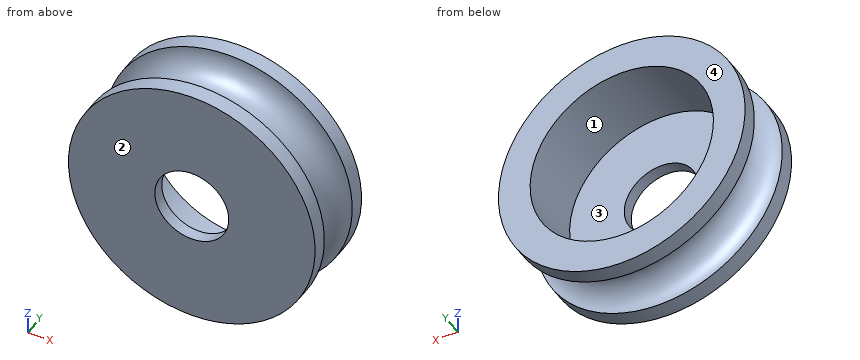
from build123d import *

# Parameters (mm, degrees)
ESBO_O1_R                = 15
RESSALTO_EXTRUS_O1_DEPTH = 10
ESBO_O9_R                = 11.15
CORTE_EXTRUS_O1_DEPTH    = 8.5
ESBO_O10_R               = 4.5
CORTE_EXTRUS_O2_DEPTH    = 24.452078799


with BuildPart() as part:
    # Esboço1 → Ressalto-extrusão1 (new body)
    with BuildSketch(Plane(origin=(0, 0, 0), x_dir=(1, 0, 0), z_dir=(0, 1, 0))):
        with Locations(Location((0, 0, 0), (0, 0, 270))):
            Circle(ESBO_O1_R)
    extrude(amount=RESSALTO_EXTRUS_O1_DEPTH)

    # Esboço8 → Corte-Revolução1 (revolve, cut)
    with BuildSketch(Plane.XY, mode=Mode.PRIVATE) as corte_revolu_o1_sk:
        with BuildLine():
            Line((15, 8), (15, 2))
            ThreePointArc((15, 2), (12, 5), (15, 8))
        make_face()
    revolve(corte_revolu_o1_sk.sketch.rotate(Axis((0, 0, 0), (0, 1, 0)), 90), axis=Axis((0, 0, 0), (0, 1, 0)), mode=Mode.SUBTRACT)

    # Esboço9 → Corte-extrusão1 (cut)
    with BuildSketch(Plane(origin=(0, 10, 0), x_dir=(1, 0, 0), z_dir=(0, 1, 0))):
        with Locations(Location((0, 0, 0), (0, 0, 270))):
            Circle(ESBO_O9_R)
    extrude(amount=-CORTE_EXTRUS_O1_DEPTH, mode=Mode.SUBTRACT)

    # Esboço10 → Corte-extrusão2 (cut, through all)
    with BuildSketch(Plane.XZ):
        with Locations(Location((0, 0, 0), (0, 0, 270))):
            Circle(ESBO_O10_R)
    extrude(amount=-CORTE_EXTRUS_O2_DEPTH, mode=Mode.SUBTRACT)


solid = part.part
The listing builds one solid part. Answer for the finished solid, in the listing's coordinates (mm). Face numbers are marked on the shaded views. A direction names the side the tool comes from. Give positions to 0.01 mm unless a question says otherwise; leave off trailing zeros. Write each loop counter-clockwise with the first axis right and the second up, starting at its lowest first coordinate (ties: lowest second). Pieces come first, ordered by that corner, then holes.
Item 1: Section B-B, the plane z = 0 is taken. Write down the section's boundary in (x, y), plus the area to 3 significant figures.
Item 2: Flat-ended cylindrical pins translate along their axes: P1, Ø1, axis at x = -8, y = 7, coming from the -Z side; P2, Ø1, axis at x = 11.5, y = 6.5, coming from the +Z side; P3, Ø14.5, axis at x = 0, z = 0, coming from the +Y side. Find the tip coordinate at first contact, or state that the pin passes through.
Item 3: Section C-C, the plane y = 9 is taken. Write down the section's boundary in (x, z).
Item 4: Section A-A, the plane x = 0 is taken. Write down the section's boundary in (y, z).
Item 5: Which of the six approach directions +Z, -Z, +X, -X, +Y, -Y give full straight-line access (tool end or side, diameter ignored) to the marked faces 3 and 4?
Item 6: Find the intervals of material crossed by line 1 along X through (y, z) = (1, 0); line 2 along Y through (x, z) = (-1.5, 11); line 3 along Z through (x, y) = (6, 2.75), in increasing order.
Item 7: Section D-D, the plane y = 4 is taken. Write down the section's boundary in (x, z).
Item 8: Determine the mould class of the marked faces 1 and 2 for opening direction X: released by +X, released by -X, zero draft, split by the parting line, or undercut.
Completed:
1. outline: (-15, 0) - (-4.5, 0) - (-4.5, 1.5) - (-11.15, 1.5) - (-11.15, 10) - (-15, 10) - (-15, 8) arc R3 cw to (-15, 2) - close; (4.5, 0) - (15, 0) - (15, 2) arc R3 cw to (15, 8) - (15, 10) - (11.15, 10) - (11.15, 1.5) - (4.5, 1.5) - close
1. area: 68.7 mm2
2. P1: stops at z = -10.75
2. P2: stops at z = 5.97
2. P3: stops at y = 1.5
3. outline: circle Ø30 at (0, 0); hole circle Ø22.3 at (0, 0)
4. outline: (0, -15) - (2, -15) arc R3 cw to (8, -15) - (10, -15) - (10, -11.15) - (1.5, -11.15) - (1.5, -4.5) - (0, -4.5) - close; (0, 4.5) - (1.5, 4.5) - (1.5, 11.15) - (10, 11.15) - (10, 15) - (8, 15) arc R3 cw to (2, 15) - (0, 15) - close
5. face 3: +Y
5. face 4: +Z, -Z, +X, -X, +Y
6. line 1: x = -15 to -4.5, 4.5 to 15
6. line 2: y = 0 to 1.5
6. line 3: z = -11.55 to -9.4, 9.4 to 11.55
7. outline: circle Ø24.34 at (0, 0); hole circle Ø22.3 at (0, 0)
8. face 1: undercut
8. face 2: zero draft
